```python
from build123d import *

# Parameters (mm, degrees)
PAD_DEPTH    = 609.6
SKETCH001_R  = 3
PAD001_DEPTH = 2.54
SKETCH002_R  = 5
PAD002_DEPTH = 2
FILLET_R     = 2


with BuildPart() as part:
    # Sketch → Pad (new body)
    with BuildSketch(Plane.XZ):
        Polygon((0, 0), (0, 16.51), (7.952592, 29.21), (0, 29.21), (0, 50.8), (2.54, 50.8), (2.54, 31.75), (12.54, 31.75), (2.54, 15.780364), (2.54, 0), align=None)
    extrude(amount=PAD_DEPTH)

    # Sketch001 (on Face4 of Pad) → Pad001 (join)
    with BuildSketch(Plane(origin=(0, 0, 0), x_dir=(0, 0, -1), z_dir=(-1, 0, 0))):
        with Locations((-44.45, 12.7)):
            Circle(SKETCH001_R)
        with Locations((-6.35, 12.7)):
            Circle(SKETCH001_R)
        with Locations((-44.45, 596.9)):
            Circle(SKETCH001_R)
        with Locations((-6.35, 596.9)):
            Circle(SKETCH001_R)
    extrude(amount=PAD001_DEPTH)

    # Sketch002 (on Face20 of Pad001) → Pad002 (join)
    with BuildSketch(Plane(origin=(-2.54, 0, 0), x_dir=(0, 0, -1), z_dir=(-1, 0, 0))):
        with Locations((-44.45, 12.7)):
            Circle(SKETCH002_R)
        with Locations((-6.35, 596.9)):
            Circle(SKETCH002_R)
        with Locations((-44.45, 596.9)):
            Circle(SKETCH002_R)
        with Locations((-6.35, 12.7)):
            Circle(SKETCH002_R)
    extrude(amount=PAD002_DEPTH)

    # Fillet
    fillet_edges = [part.edges().sort_by_distance(p)[0] for p in [
        (0, -304.8, 29.21),
        (0, -304.8, 16.51),
        (12.54, -304.8, 31.75),
        (7.952592, -304.8, 29.21),
    ]]
    fillet(fillet_edges, radius=FILLET_R)


solid = part.part
```
For this review, take the finished solid that the model builds, in its own axes (mm). A direction names the side the tool comes from. Coordinates: 2 decimals unless noted, no trailing zeros. Loops run counter-clockwise (first coordinate to the right, second up) from the corner with the lowest first, then second, coordinate; pieces in that order, holes last.
1. Insertion check: P1, Ø1, axis at y = -527.5, z = 20.5, coming from the +X side; P2, Ø12.5, axis at y = -234, z = 8.5, coming from the -X side; P3, Ø21, axis at y = -435.5, z = 45, coming from the +X side; P4, Ø3, axis at x = -2, y = -101.5, coming from the +Z side. Each pin has a flat end and moves straight along its axis. Give the tip position at first contact, or say it passes through.
2. Mouldability with a two-part tool opening along Z and no side actions: class faces 1 (the flat face through (2.54, -301, 8)), 2 (the flat face through (6.638, -300.533, 22.325)), 3 (the flat face through (-2.54, -13, 3)) as +Z half, -Z half, draft (parallel to the pull), parting line (faces both ways), or undercut.
3. For line 1 (X direction, y = -34.5, z = 37); line 2 (X direction, y = -256.5, z = 22); line 3 (Z direction, x = 5.5, y = -487), list the stretches that pass through material, from the lowest coordinate up.
4. For faces 4 (the flat face through (2.54, -301, 41)), 5 (the flat face through (-2.54, -597, 41)), 6 (the flat face through (5.9, 0, 25.5)), 7 (the flat face through (-4.54, -597, 45)), 8 (the cylindrical face through (-3.526, -601.857, 45.101)), list the 3-axis set-ups (+Z, -Z, +X, -X, +Y, -Y) from which the entire face can be reached by the end or side of a thin tool; tool diameter is ignored.
5. Add section A-A, the plane y = -162. Give the boundary of the cut face in (x, z).
Result:
1. P1: stops at x = 5.81
1. P2: stops at x = 0
1. P3: stops at x = 2.54
1. P4: passes through
2. face 1: draft
2. face 2: -Z half
2. face 3: undercut
3. line 1: x = 0 to 2.54
3. line 2: x = 3.44 to 6.43
3. line 3: z = 20.51 to 25.29, 28.84 to 31.75
4. face 4: +Z, +X, +Y, -Y
4. face 5: none
4. face 6: +Z, -Z, +X, -X, +Y
4. face 7: +Z, -Z, -X, +Y, -Y
4. face 8: -X
5. outline: (0, 0) - (2.54, 0) - (2.54, 15.78) - (10.62, 28.69) arc R2 ccw to (8.93, 31.75) - (2.54, 31.75) - (2.54, 50.8) - (0, 50.8) - (0, 31.21) arc R2 ccw to (2, 29.21) - (4.34, 29.21) arc R2 cw to (6.04, 26.15) - (0.3, 17) arc R2 ccw to (0, 15.94) - close
